Source: CAD feature listing. Evaluate the final solid. Frame: model axes, mm. Face numbers are marked on the shaded views. A direction names the side the tool comes from. Coordinates: 2 decimals unless noted, no trailing zeros. Loops run counter-clockwise (first coordinate to the right, second up) from the corner with the lowest first, then second, coordinate; pieces in that order, holes last. Notation, with made-up numbers: (-37.75, -7.75) - (1.25, -7.75) arc R23 cw to (1.25, 19.25) - close; hole circle Ø6 at (7.25, -33.5). An arc over 180 degrees is marked (long way). Use one line per item in the form item = value. Start each with the question number.
from build123d import *

# Parameters (mm, degrees)
SKETCH2_W           = 100
SKETCH2_H           = 65
BOSS_EXTRUDE1_DEPTH = 50
FILLET1_R           = 10
SHELL1_T            = -5
SKETCH3_R           = 5
CUT_EXTRUDE1_DEPTH  = 101


with BuildPart() as part:
    # Sketch2 → Boss-Extrude1 (new body)
    with BuildSketch(Plane.XY):
        with Locations((50, 32.5)):
            Rectangle(SKETCH2_W, SKETCH2_H)
    extrude(amount=BOSS_EXTRUDE1_DEPTH)

    # Fillet1
    fillet1_edges = [part.edges().sort_by_distance(p)[0] for p in [
        (100, 32.5, 50),
        (0, 32.5, 50),
        (100, 32.5, 0),
        (0, 32.5, 0),
    ]]
    fillet(fillet1_edges, radius=FILLET1_R)

    # Shell1
    shell1_openings = [part.faces().sort_by_distance(p)[0] for p in [
        (50, 65, 25),
    ]]
    offset(amount=SHELL1_T, openings=shell1_openings, kind=Kind.INTERSECTION)

    # Sketch3 → Cut-Extrude1 (cut, through all)
    with BuildSketch(Plane(origin=(100, 0, 0), x_dir=(0, 0, -1), z_dir=(1, 0, 0))):
        with Locations((-25, 40)):
            Circle(SKETCH3_R)
    extrude(amount=-CUT_EXTRUDE1_DEPTH, mode=Mode.SUBTRACT)


solid = part.part
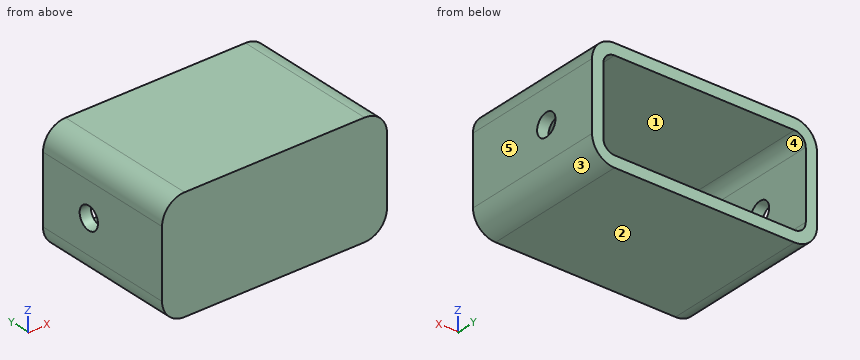
(1) Cut plane D-D, the plane y = 23. Output: boundary loops of the cut face in (x, z), plus the area to 3 significant figures.
(2) Contact query for flat-ended pins moving along their axis: pin 1 (9 mm diameter, centred on y = 40, z = 25, fed in from +X); pin 2 (2 mm diameter, centred on x = 30, z = 37, fed in from -Y). Output: stop coordinate, or through.
(3) Cut plane B-B, the plane y = 43. Output: boundary loops of the cut face in (x, z).
(4) Access query for the marked faces 4 and 5. Directions: +Z, -Z, +X, -X, +Y, -Y. A direction counts if a zero-diameter tool reaches every point of the face in a straight line with its end or side. Return the directions, or none.
(5) Cut plane A-A, the plane z = 25. Output: boundary loops of the cut face in (x, y), plus the area to 3 significant figures.
(6) Mould query, pull axis X, two halves, no side actions, for the marked faces 1, 2 and 3. Classes: +X half, -X half, draft (parallel to the pull), parting line (faces both ways), or undercut.
(7) Cut plane C-C, the plane x = 72. Output: boundary loops of the cut face in (y, z), plus the area to 3 significant figures.
(8) Material intervals for line 1 (Y direction, x = 2.15, z = 25); line 2 (Z direction, x = 28, y = 19); line 3 (X direction, y = 24, z = 36), sorted ascending.
Recorded:
q1.outline = (0, 10) arc R10 ccw to (10, 0) - (90, 0) arc R10 ccw to (100, 10) - (100, 40) arc R10 ccw to (90, 50) - (10, 50) arc R10 ccw to (0, 40) - close; hole (5, 10) arc R5 ccw to (10, 5) - (90, 5) arc R5 ccw to (95, 10) - (95, 40) arc R5 ccw to (90, 45) - (10, 45) arc R5 ccw to (5, 40) - close
q1.area = 1,340 mm²
q2.pin_1 = through
q2.pin_2 = 0
q3.outline = (0, 10) arc R10 ccw to (10, 0) - (90, 0) arc R10 ccw to (100, 10) - (100, 21) - (95, 21) - (95, 10) arc R5 cw to (90, 5) - (10, 5) arc R5 cw to (5, 10) - (5, 21) - (0, 21) - close; (0, 29) - (5, 29) - (5, 40) arc R5 cw to (10, 45) - (90, 45) arc R5 cw to (95, 40) - (95, 29) - (100, 29) - (100, 40) arc R10 ccw to (90, 50) - (10, 50) arc R10 ccw to (0, 40) - close
q4.face_4 = +Y
q4.face_5 = +Z, -Z, +X, +Y, -Y
q5.outline = (0, 0) - (100, 0) - (100, 35) - (95, 35) - (95, 5) - (5, 5) - (5, 35) - (0, 35) - close; (0, 45) - (5, 45) - (5, 65) - (0, 65) - close; (95, 45) - (100, 45) - (100, 65) - (95, 65) - close
q5.area = 1,000 mm²
q6.face_1 = undercut
q6.face_2 = draft
q6.face_3 = +X half
q7.outline = (0, 0) - (65, 0) - (65, 5) - (5, 5) - (5, 45) - (65, 45) - (65, 50) - (0, 50) - close
q7.area = 850 mm²
q8.line_1 = 0 to 35, 45 to 65
q8.line_2 = 0 to 5, 45 to 50
q8.line_3 = 0 to 5, 95 to 100
